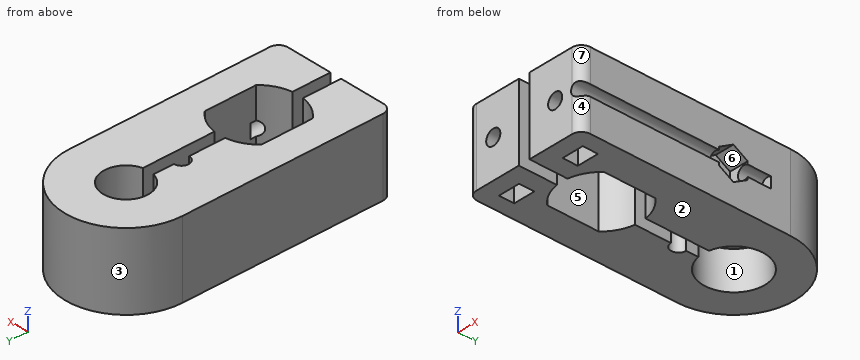
```python
from build123d import *

# Parameters (mm, degrees)
PAD001_DEPTH    = 20
SKETCH012_R     = 1.75
POCKET008_DEPTH = 50
POCKET009_DEPTH = 5
POCKET010_DEPTH = 15
SKETCH015_R     = 2
POCKET011_DEPTH = 15
SKETCH016_R     = 8.1
POCKET012_DEPTH = 10


with BuildPart() as part:
    # Sketch011 → Pad001 (new body)
    with BuildSketch(Plane.XY):
        with BuildLine():
            Line((-8, -28.1), (-8, -41.6))
            ThreePointArc((-8, -41.6), (-5.061117, -43.925857), (-1.5, -45.094227))
            Line((-1.5, -55.094227), (-1.5, -45.094227))
            Line((-13.5, -55.094227), (-1.5, -55.094227))
            ThreePointArc((-16, -52.594227), (-15.267767, -54.361994), (-13.5, -55.094227))
            Line((-16, 0), (-16, -52.594227))
            ThreePointArc((16, 0), (0, 16), (-16, 0))
            Line((16, -52.594227), (16, 0))
            ThreePointArc((13.5, -55.094227), (15.267767, -54.361994), (16, -52.594227))
            Line((1.5, -55.094227), (13.5, -55.094227))
            Line((1.5, -55.094227), (1.5, -45.094227))
            ThreePointArc((1.5, -45.094227), (5.061117, -43.925857), (8, -41.6))
            Line((8, -41.6), (8, -28.1))
            ThreePointArc((8, -28.1), (5.061117, -25.774143), (1.5, -24.605773))
            Line((1.5, -5.809475), (1.5, -24.605773))
            ThreePointArc((1.5, -5.809475), (0, 6), (-1.5, -5.809475))
            Line((-1.5, -5.809475), (-1.5, -11.150936))
            ThreePointArc((-1.5, -11.150936), (-3.5, -13.150936), (-1.5, -15.150936))
            Line((-1.5, -15.150936), (-1.5, -24.605773))
            ThreePointArc((-1.5, -24.605773), (-5.061117, -25.774143), (-8, -28.1))
        make_face()
    extrude(amount=PAD001_DEPTH)

    # Sketch012 (on Face9 of Pad001) → Pocket008 (cut)
    with BuildSketch(Plane.XZ.offset(55.094227)):
        with Locations((15, 10)):
            Circle(SKETCH012_R)
    extrude(amount=-POCKET008_DEPTH, mode=Mode.SUBTRACT)

    # Sketch013 (on Face17 of Pocket008) → Pocket009 (cut)
    with BuildSketch(Plane(origin=(16, 0, 0), x_dir=(0, -1, 0), z_dir=(-1, 0, 0))):
        Polygon((18.75, 7.834936), (18.75, 12.165064), (15, 14.330127), (11.25, 12.165064), (11.25, 7.834936), (15, 5.669873), align=None)
    extrude(amount=POCKET009_DEPTH, mode=Mode.SUBTRACT)

    # Sketch014 → Pocket010 (cut)
    with BuildSketch(Plane(origin=(0, 0, 0), x_dir=(1, 0, 0), z_dir=(0, 0, -1))):
        Polygon((-7, 50.72662), (-6.15, 50.72662), (-6.15, 46.72662), (-11.85, 46.72662), (-11.85, 50.72662), (-11, 50.72662), align=None)
        Polygon((11, 50.72662), (11.85, 50.72662), (11.85, 46.72662), (6.15, 46.72662), (6.15, 50.72662), (7, 50.72662), align=None)
    extrude(amount=-POCKET010_DEPTH, mode=Mode.SUBTRACT)

    # Sketch015 (on Face19 of Pocket010) → Pocket011 (cut)
    with BuildSketch(Plane.XZ.offset(55.094227)):
        with Locations((-8.75, 10)):
            Circle(SKETCH015_R)
        with Locations((8.75, 10)):
            Circle(SKETCH015_R)
    extrude(amount=-POCKET011_DEPTH, mode=Mode.SUBTRACT)

    # Sketch016 (on Face4 of Pocket011) → Pocket012 (cut)
    with BuildSketch(Plane(origin=(0, 0, 0), x_dir=(1, 0, 0), z_dir=(0, 0, -1))):
        Circle(SKETCH016_R)
    extrude(amount=-POCKET012_DEPTH, mode=Mode.SUBTRACT)


solid = part.part
```
Input: part model. Units: mm. Frame: model coordinates. Face numbers are marked on the shaded views. A direction names the side the tool comes from. Give positions to 0.01 mm unless a question says otherwise; leave off trailing zeros. Write each loop counter-clockwise with the first axis right and the second up, starting at its lowest first coordinate (ties: lowest second). Pieces come first, ordered by that corner, then holes. Notation, with made-up numbers: (58, -14) - (74, -14) arc R11 cw to (74, 0) - close; hole circle Ø6 at (-38.5, 31.5). An arc over 180 degrees is marked (long way). Write item = value, one per line. Start each with the question number.
1) Cut plane C-C (z = 4). Return loops of the section in (x, y).
2) Draft query along X for the marked faces 1, 2, 3 and 4. Return one class per face: pulls with the +X half, pulls with the -X half, needs draft (parallel to the pull), parting line crosses it, or undercut.
3) Pin query (flat end, axial travel): pin 1 (6 mm diameter, centred on x = 9.5, z = 15.5, fed in from +Y); pin 2 (1.2 mm diameter, centred on x = 8.5, y = -48.5, fed in from -Z); pin 3 (9.5 mm diameter, centred on x = 0, y = 0, fed in from -Z); pin 4 (3 mm diameter, centred on x = 8.75, z = 10, fed in from +Y). Return the tip coordinate at first contact, or that it passes through.
4) Cut plane A-A (z = 18.25). Return loops of the section in (x, y), and give its area (3 significant figures).
5) Cut plane B-B (x = 0). Return loops of the section in (y, z).
6) Material intervals for L1, parallel to X at y = -11, z = 14.5; L2, parallel to X at y = -50, z = 14.75; L3, parallel to X at y = -44.25, z = 10, sorted ascending. Write a range as [from, to].
7) Reachability of the marked faces 5, 6 and 7 from +Z, -Z, +X, -X, +Y, -Y: full face, straight path, thin tool, end or side. Return the list, or none.
8) Cut plane D-D (x = 8.75). Return loops of the section in (y, z), and give its area (3 significant figures).
Answers follow:
q1.outline = (-16, -52.59) arc R2.5 ccw to (-13.5, -55.09) - (-1.5, -55.09) - (-1.5, -45.09) arc R10.69 cw to (-8, -41.6) - (-8, -28.1) arc R10.69 cw to (-1.5, -24.61) - (-1.5, -15.15) arc R2 cw to (-1.5, -11.15) - (-1.5, -7.96) arc R8.1 cw (long way) to (1.5, -7.96) - (1.5, -24.61) arc R10.69 cw to (8, -28.1) - (8, -41.6) arc R10.69 cw to (1.5, -45.09) - (1.5, -55.09) - (13.5, -55.09) arc R2.5 ccw to (16, -52.59) - (16, 0) arc R16 ccw to (-16, 0) - close; hole (-11.85, -50.73) - (-6.15, -50.73) - (-6.15, -46.73) - (-11.85, -46.73) - close; hole (6.15, -50.73) - (11.85, -50.73) - (11.85, -46.73) - (6.15, -46.73) - close
q2.face_1 = undercut
q2.face_2 = needs draft
q2.face_3 = parting line crosses it
q2.face_4 = pulls with the +X half
q3.pin_1 = 14.62
q3.pin_2 = 15
q3.pin_3 = through
q3.pin_4 = 14.26
q4.outline = (-16, -52.59) arc R2.5 ccw to (-13.5, -55.09) - (-1.5, -55.09) - (-1.5, -45.09) arc R10.69 cw to (-8, -41.6) - (-8, -28.1) arc R10.69 cw to (-1.5, -24.61) - (-1.5, -15.15) arc R2 cw to (-1.5, -11.15) - (-1.5, -5.81) arc R6 cw (long way) to (1.5, -5.81) - (1.5, -24.61) arc R10.69 cw to (8, -28.1) - (8, -41.6) arc R10.69 cw to (1.5, -45.09) - (1.5, -55.09) - (13.5, -55.09) arc R2.5 ccw to (16, -52.59) - (16, 0) arc R16 ccw to (-16, 0) - close
q4.area = 1,660 mm^2
q5.outline = (6, 10) - (8.1, 10) - (8.1, 0) - (16, 0) - (16, 20) - (6, 20) - close
q6.L1 = [-16, -1.5], [1.5, 16]
q6.L2 = [-16, -11.85], [-6.15, -1.5], [1.5, 6.15], [11.85, 16]
q6.L3 = [-16, -10.75], [-6.75, -4.41], [4.41, 6.75], [10.75, 13.25]
q7.face_5 = +Z, -Z
q7.face_6 = +X
q7.face_7 = +Z, -Z, +X, -Y
q8.outline = (-55.09, 0) - (-50.73, 0) - (-50.73, 8) - (-55.09, 8) - close; (-55.09, 12) - (-50.73, 12) - (-50.73, 15) - (-46.73, 15) - (-46.73, 12) - (-40.09, 12) - (-40.09, 8) - (-46.73, 8) - (-46.73, 0) - (13.4, 0) - (13.4, 20) - (-55.09, 20) - close
q8.area = 1,270 mm^2
